from build123d import *

# Parameters (mm, degrees)
EXTRUDE_1_DEPTH     = 3
SKETCH_1_3_R        = 2.25
EXTRUDE_2_DEPTH     = 10
SKETCH_2_W          = 5
SKETCH_2_H          = 2
CUT_EXTRUDE_1_DEPTH = 2


with BuildPart() as part:
    # Sketch 1 → Extrude 1 (new body)
    with BuildSketch(Plane.XY):
        with BuildLine():
            ThreePointArc((0, 2.25), (-2.25, 0), (0, -2.25))
            Line((0, -2.25), (50, -2.25))
            ThreePointArc((50, -2.25), (52.25, 0), (50, 2.25))
            Line((50, 2.25), (0, 2.25))
        make_face()
    extrude(amount=EXTRUDE_1_DEPTH)

    # Sketch 1_3 → Extrude 2 (add)
    with BuildSketch(Plane.XY):
        with Locations(Location((0, 0, 0), (0, 0, 270))):
            Circle(SKETCH_1_3_R)
        with Locations(Location((50, 0, 0), (0, 0, 90))):
            Circle(SKETCH_1_3_R)
    extrude(amount=EXTRUDE_2_DEPTH)

    # Sketch 2 → Cut-Extrude 1 (cut)
    with BuildSketch(Plane.XY.offset(10)):
        Rectangle(SKETCH_2_W, SKETCH_2_H)
        with Locations((50, 0)):
            Rectangle(SKETCH_2_W, SKETCH_2_H)
    extrude(amount=-CUT_EXTRUDE_1_DEPTH, mode=Mode.SUBTRACT)


solid = part.part
The listing builds one solid part. Answer for the finished solid, in the listing's coordinates (mm). A direction names the side the tool comes from. Round coordinates to 2 decimals unless told otherwise and drop trailing zeros. Order: outer loops, then holes, each group sorted by start corner. A loop starts at its lowest first (then second) coordinate and runs counter-clockwise, first axis right, second up. Notation, with made-up numbers: M 44.25,-27.75 L 96.25,-27.75 A30 cw 96.25,7.25 Z; hole C 14,27 d2. An arc over 180 degrees is marked long. Answer in a Markdown table with one row per item. Add a question column.
1) The part is cut by section B-B on y = 0. Determine the outline of the cut face in (x, z), plus the area to 4 significant figures.
2) The part is cut by section D-D on z = 2. Determine the outline of the cut face in (x, y), plus the area to 3 significant figures.
3) Which of the six approach directions +Z, -Z, +X, -X, +Y, -Y give full straight-line access (tool end or side, diameter ignored) to faces 1 (the face through (0, 1, 9)), 2 (the face through (25, -2.25, 1))?
4) Determine the mould class of faces 3 (the face through (25, 2.25, 1)), 4 (the face through (25, 0, 3)) for opening direction X: pulls with the +X half, pulls with the -X half, needs draft (parallel to the pull), parting line crosses it, or undercut.
5) Consider line 1 along Z through (x, y) = (30, -0.6); line 2 along X through (y, z) = (1.15, 8.75); line 3 along X through (y, z) = (1.45, 4.75). Determine where each line is inside the solid, lowest interval first. Write a range as from..to.
6) The part is cut by section A-A on z = 8.5. Determine the outline of the cut face in (x, y), plus the area to 3 significant figures.
7) The part is cut by section C-C on z = 4. Determine the outline of the cut face in (x, y), plus the area to 3 significant figures.
8) Flat-ended cylindrical pins translate along their axes: pin 1 Ø1.6 at (x, y) = (49, 0) entering from +Z; pin 2 Ø1 at (x, y) = (30.5, -0.5) entering from +Z; pin 3 Ø0.6 at (x, z) = (49.5, 9) entering from +Y. Find the tip coordinate at first contact, or state that the pin passes through.
Findings below:
| question | item | result |
|---|---|---|
| 1 | outline | M -2.25,0 L 52.25,0 L 52.25,8 L 47.75,8 L 47.75,3 L 2.25,3 L 2.25,8 L -2.25,8 Z |
| 1 | area | 208.5 mm² |
| 2 | outline | M 0,-2.25 L 50,-2.25 A2.25 ccw 50,2.25 L 0,2.25 A2.25 ccw Z |
| 2 | area | 241 mm² |
| 3 | face 1 | +Z, +X, -X |
| 3 | face 2 | +Z, -Z, +X, -X, -Y |
| 4 | face 3 | needs draft |
| 4 | face 4 | undercut |
| 5 | line 1 | z = 0..3 |
| 5 | line 2 | x = -1.93..1.93, 48.07..51.93 |
| 5 | line 3 | x = -1.72..1.72, 48.28..51.72 |
| 6 | outline | M -2.02,-1 A2.25 ccw 2.02,-1 Z; M -2.02,1 L 2.02,1 A2.25 ccw Z; M 47.98,-1 A2.25 ccw 52.02,-1 Z; M 47.98,1 L 52.02,1 A2.25 ccw Z |
| 6 | area | 14.4 mm² |
| 7 | outline | C 0,0 d4.5; C 50,0 d4.5 |
| 7 | area | 31.8 mm² |
| 8 | pin 1 | stops at z = 8 |
| 8 | pin 2 | stops at z = 3 |
| 8 | pin 3 | stops at y = 2.24 |
